Verification items for the finished model (mm, model axes). Round coordinates to 2 decimals unless told otherwise and drop trailing zeros. Write each loop counter-clockwise with the first axis right and the second up, starting at its lowest first coordinate (ties: lowest second). Pieces come first, ordered by that corner, then holes. Notation, with made-up numbers: (79, 12) -> (135, 12) arc R23 cw to (135, 48) -> close; hole circle Ø3 at (47, -22). An arc over 180 degrees is marked (long way). Answer as a JSON object with one key per item and string values. Group by question number.
(1) Sectioned sample at B-B on z = 6.5. Record the cut outline in (x, y).
(2) Sectioned sample at A-A on y = 0.9. Count the separate pieces of the cut face and the enclosed holes in it, and give its area (3 significant figures).
(3) Scan lines: L1, parallel to X at y = 2.8, z = 82.55; L2, parallel to X at y = 3.95, z = 38.1; L3, parallel to Z at x = 10.5, y = 1.8. Record each from-to range of solid material in increasing order. Write a range as from..to.
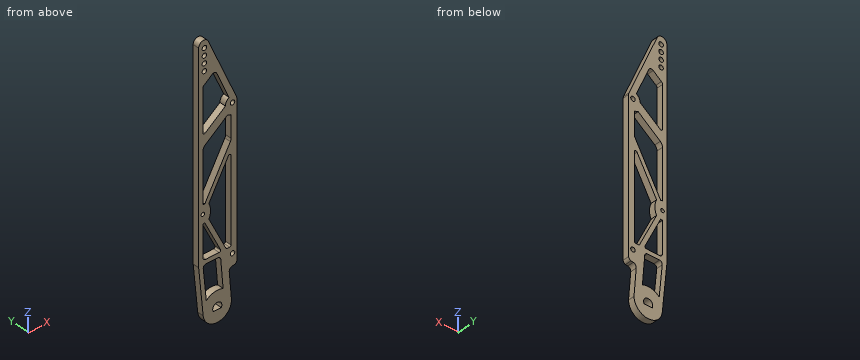
```python
from build123d import *

# Parameters (mm, degrees)
SKETCH2_R           = 2
SKETCH2_R_2         = 1.5875
SKETCH2_R_3         = 1.999999991
BOSS_EXTRUDE1_DEPTH = 5.588


with BuildPart() as part:
    # Sketch2 → Boss-Extrude1 (new body)
    with BuildSketch(Plane(origin=(0, 0, 0), x_dir=(1, 0, 0), z_dir=(0, 1, 0))):
        with BuildLine():
            ThreePointArc((17.295902343, -30.526810701), (16.688093876, -28.878103365), (15.15555913, -28.018449791))
            Line((15.15555913, -28.018449791), (13.238676936, -27.713033224))
            ThreePointArc((13.238676936, -27.713033224), (11.241051513, -26.538356195), (10.573787778, -24.319092227))
            Line((10.573787778, -24.319092227), (12.5603, 0))
            ThreePointArc((12.5603, 0), (0.603657177, 12.545785512), (-12.502275592, 1.2059192))
            Line((-12.502275592, 1.2059192), (-16.498266045, -40.222207921))
            ThreePointArc((-16.498266045, -40.222207921), (-16.507064815, -40.344000039), (-16.51, -40.466074291))
            Line((-16.51, -40.466074291), (-16.51, -221.328861788))
            ThreePointArc((-16.51, -221.328861788), (-12.970187584, -225.680718913), (-7.988667969, -223.101301399))
            Line((-7.988667969, -223.101301399), (16.979901226, -165.677523619))
            ThreePointArc((16.979901226, -165.677523619), (17.216065593, -164.934164738), (17.295902343, -164.158289667))
            Line((17.295902343, -164.158289667), (17.295902343, -30.526810701))
        make_face()
        with Locations(Location((-11.43, -219.075, 0), (0, 0, 270))):
            Circle(SKETCH2_R, mode=Mode.SUBTRACT)
        with Locations(Location((-11.43, -212.725, 0), (0, 0, 270))):
            Circle(SKETCH2_R, mode=Mode.SUBTRACT)
        with Locations(Location((-11.43, -206.375, 0), (0, 0, 270))):
            Circle(SKETCH2_R, mode=Mode.SUBTRACT)
        with Locations(Location((-11.43, -200.025, 0), (0, 0, 270))):
            Circle(SKETCH2_R, mode=Mode.SUBTRACT)
        with BuildLine():
            ThreePointArc((7.135902343, -162.410770806), (8.023611961, -165.648962244), (10.438542905, -167.981776143))
            Line((10.438542905, -167.981776143), (-0.534170778, -193.217289931))
            ThreePointArc((-0.534170778, -193.217289931), (-2.234040931, -194.665234867), (-4.420389569, -194.211381682))
            Line((-4.420389569, -194.211381682), (-11.716886202, -188.551043102))
            ThreePointArc((-11.716886202, -188.551043102), (-12.441018517, -187.661516081), (-12.7, -186.544128716))
            Line((-12.7, -186.544128716), (-12.7, -149.615408258))
            ThreePointArc((-12.7, -149.615408258), (-11.988693683, -148.474898999), (-10.651556899, -148.611951065))
            Line((-10.651556899, -148.611951065), (7.135902343, -162.410770806))
        make_face(mode=Mode.SUBTRACT)
        with BuildLine():
            ThreePointArc((12.215902343, -152.970817152), (10.520298026, -153.359206519), (8.923603828, -154.049487576))
            Line((8.923603828, -154.049487576), (-10.733772403, -138.80005889))
            ThreePointArc((-10.733772403, -138.80005889), (-12.182037035, -137.021004847), (-12.7, -134.786230117))
            Line((-12.7, -134.786230117), (-12.7, -90.4875))
            ThreePointArc((-12.7, -90.4875), (-11.888769677, -90.445936399), (-11.086035141, -90.321680879))
            Line((-11.086035141, -90.321680879), (11.575760855, -131.079432803))
            ThreePointArc((11.575760855, -131.079432803), (12.053263487, -132.272915946), (12.215902343, -133.548047069))
            Line((12.215902343, -133.548047069), (12.215902343, -152.970817152))
        make_face(mode=Mode.SUBTRACT)
        with Locations(Location((13.485902343, -162.410770806, 0), (0, 0, 270))):
            Circle(SKETCH2_R, mode=Mode.SUBTRACT)
        with Locations(Location((-12.7, -82.55, 0), (0, 0, 270))):
            Circle(SKETCH2_R_2, mode=Mode.SUBTRACT)
        with BuildLine():
            Line((-10.16, -44.337182032), (1.663048834, -44.337182032))
            ThreePointArc((1.663048834, -44.337182032), (2.739129831, -44.932682449), (2.806066447, -46.160725831))
            Line((2.806066447, -46.160725831), (-11.055993219, -74.784618621))
            ThreePointArc((-11.055993219, -74.784618621), (-11.873503915, -74.655646925), (-12.7, -74.6125))
            Line((-12.7, -74.6125), (-12.7, -46.877182032))
            ThreePointArc((-12.7, -46.877182032), (-11.956051224, -45.081130808), (-10.16, -44.337182032))
        make_face(mode=Mode.SUBTRACT)
        with BuildLine():
            ThreePointArc((-9.903213406, -40.527182032), (-11.783508673, -39.694838236), (-12.431479451, -37.743315662))
            Line((-12.431479451, -37.743315662), (-9.755434212, -9.99962016))
            ThreePointArc((-9.755434212, -9.99962016), (-2.756273581, -13.695395429), (5.127655889, -12.99492382))
            Line((5.127655889, -12.99492382), (3.069264048, -38.19397392))
            ThreePointArc((3.069264048, -38.19397392), (2.259083254, -39.854914801), (0.537695935, -40.527182032))
            Line((0.537695935, -40.527182032), (-9.903213406, -40.527182032))
        make_face(mode=Mode.SUBTRACT)
        with BuildLine():
            Line((-3.521718331, 2), (3.521718331, 2))
            ThreePointArc((3.521718331, 2), (0, -4.05), (-3.521718331, 2))
        make_face(mode=Mode.SUBTRACT)
        with BuildLine():
            ThreePointArc((-7.44734835, -89.025591197), (-5.976040897, -82.55), (-7.44734835, -76.074408803))
            Line((-7.44734835, -76.074408803), (7.575478058, -45.053638233))
            ThreePointArc((7.575478058, -45.053638233), (8.043996088, -44.531101035), (8.718495671, -44.337182032))
            Line((8.718495671, -44.337182032), (10.945902343, -44.337182032))
            ThreePointArc((10.945902343, -44.337182032), (11.843927955, -44.70915642), (12.215902343, -45.607182032))
            Line((12.215902343, -45.607182032), (12.215902343, -119.492817968))
            ThreePointArc((12.215902343, -119.492817968), (11.264685124, -120.722158254), (9.835937715, -120.109971535))
            Line((9.835937715, -120.109971535), (-7.44734835, -89.025591197))
        make_face(mode=Mode.SUBTRACT)
        with Locations(Location((13.485902343, -38.1, 0), (0, 0, 270))):
            Circle(SKETCH2_R_3, mode=Mode.SUBTRACT)
    extrude(amount=BOSS_EXTRUDE1_DEPTH)


solid = part.part
```
Computed values:
{
 "1": {"outline": "(-13.25, 0) -> (12.03, 0) -> (12.03, 5.59) -> (-13.25, 5.59) -> close"},
 "2": {"separate pieces": "1", "enclosed holes": "13", "area": "3,430 mm2"},
 "3": {"L1": "-16.51..-14.29, -11.11..-5.98, 12.22..17.3", "L2": "-16.29..-12.44, 3.08..11.49, 15.49..17.3", "L3": "-6.89..44.34, 120.68..129.14, 153.37..180.58"}
}
